Geometry: final body of the model. Coordinates: model frame, mm. Face numbers are marked on the shaded views. A direction names the side the tool comes from. Coordinates: 2 decimals unless noted, no trailing zeros. Order: outer loops, then holes, each group sorted by start corner. A loop starts at its lowest first (then second) coordinate and runs counter-clockwise, first axis right, second up. Notation, with made-up numbers: (-21, -16) - (10, -16) arc R17 ccw to (10, 13) - close; hole circle Ø9 at (9, 68). An arc over 180 degrees is marked (long way). Use a Markdown table: item, result. Add a question column.
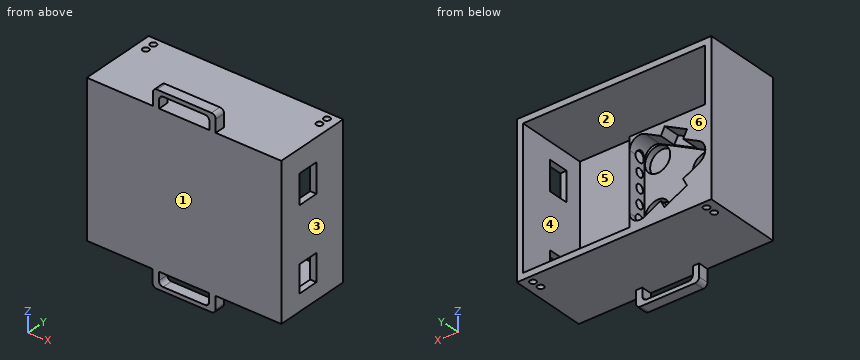
```python
from build123d import *

# Parameters (mm, degrees)
SKETCH1_W           = 92.7
SKETCH1_H           = 37
BOSS_EXTRUDE1_DEPTH = 72
SKETCH3_W           = 86.7
SKETCH3_H           = 66
CUT_EXTRUDE1_DEPTH  = 34
SKETCH6_W           = 13
SKETCH6_H           = 10
SKETCH6_W_2         = 14
CUT_EXTRUDE2_DEPTH  = 3
SKETCH8_W           = 30
SKETCH8_H           = 5
BOSS_EXTRUDE2_DEPTH = 8
SKETCH9_W           = 24
SKETCH9_H           = 6
CUT_EXTRUDE3_DEPTH  = 8
FILLET3_R           = 2
FILLET4_R           = 2
SKETCH10_W          = 30
SKETCH10_H          = 5
BOSS_EXTRUDE3_DEPTH = 8
SKETCH11_W          = 24
SKETCH11_H          = 6
CUT_EXTRUDE4_DEPTH  = 8
FILLET5_R           = 2
BOSS_EXTRUDE4_DEPTH = 40
CUT_EXTRUDE5_DEPTH  = 9
SKETCH15_R          = 6
CUT_EXTRUDE6_DEPTH  = 12
CUT_EXTRUDE7_DEPTH  = 8
SKETCH26_R          = 2.5
SKETCH26_R_2        = 2
CUT_EXTRUDE8_DEPTH  = 1


with BuildPart() as part:
    # Sketch1 → Boss-Extrude1 (new body)
    with BuildSketch(Plane.XY):
        with Locations((46.35, 18.5)):
            Rectangle(SKETCH1_W, SKETCH1_H)
    extrude(amount=-BOSS_EXTRUDE1_DEPTH)

    # Sketch3 → Cut-Extrude1 (cut)
    with BuildSketch(Plane(origin=(0, 37, 0), x_dir=(1, 0, 0), z_dir=(0, 1, 0))):
        with Locations((46.35, 36)):
            Rectangle(SKETCH3_W, SKETCH3_H)
    extrude(amount=-CUT_EXTRUDE1_DEPTH, mode=Mode.SUBTRACT)

    # Sketch6 → Cut-Extrude2 (cut)
    with BuildSketch(Plane(origin=(92.7, 0, 0), x_dir=(0, 0, -1), z_dir=(1, 0, 0))):
        with Locations((57.5, 16)):
            Rectangle(SKETCH6_W, SKETCH6_H)
        with Locations((18, 16)):
            Rectangle(SKETCH6_W_2, SKETCH6_H)
    extrude(amount=-CUT_EXTRUDE2_DEPTH, mode=Mode.SUBTRACT)

    # Sketch8 → Boss-Extrude2 (add)
    with BuildSketch(Plane.XY):
        with Locations((46.447728755, 2.5)):
            Rectangle(SKETCH8_W, SKETCH8_H)
    extrude(amount=BOSS_EXTRUDE2_DEPTH)

    # Sketch9 → Cut-Extrude3 (cut)
    with BuildSketch(Plane(origin=(0, 5, 0), x_dir=(1, 0, 0), z_dir=(0, 1, 0))):
        with Locations((46.447728755, -3)):
            Rectangle(SKETCH9_W, SKETCH9_H)
    extrude(amount=-CUT_EXTRUDE3_DEPTH, mode=Mode.SUBTRACT)

    # Fillet3
    fillet3_edges = [part.edges().sort_by_distance(p)[0] for p in [
        (31.447728755, 2.5, 8),
        (61.447728755, 2.5, 8),
    ]]
    fillet(fillet3_edges, radius=FILLET3_R)

    # Fillet4
    fillet4_edges = [part.edges().sort_by_distance(p)[0] for p in [
        (58.447728755, 2.5, 6),
        (34.447728755, 2.5, 6),
    ]]
    fillet(fillet4_edges, radius=FILLET4_R)

    # Sketch10 → Boss-Extrude3 (add)
    with BuildSketch(Plane(origin=(0, 0, -72), x_dir=(-1, 0, 0), z_dir=(0, 0, -1))):
        with Locations((-46.35, 2.5)):
            Rectangle(SKETCH10_W, SKETCH10_H)
    extrude(amount=BOSS_EXTRUDE3_DEPTH)

    # Sketch11 → Cut-Extrude4 (cut)
    with BuildSketch(Plane(origin=(0, 5, 0), x_dir=(1, 0, 0), z_dir=(0, 1, 0))):
        with Locations((46.35, 75)):
            Rectangle(SKETCH11_W, SKETCH11_H)
    extrude(amount=-CUT_EXTRUDE4_DEPTH, mode=Mode.SUBTRACT)

    # Fillet5
    fillet5_edges = [part.edges().sort_by_distance(p)[0] for p in [
        (61.35, 2.5, -80),
        (31.35, 2.5, -80),
        (34.35, 2.5, -78),
        (58.35, 2.5, -78),
    ]]
    fillet(fillet5_edges, radius=FILLET5_R)

    # Sketch13 → Boss-Extrude4 (add)
    with BuildSketch(Plane.XY.offset(-69)):
        Polygon((3, 37), (3, 25), (16, 25), (16, 26), (26, 26), (26, 25), (39, 25), (39, 37), align=None)
    extrude(amount=BOSS_EXTRUDE4_DEPTH)

    # Sketch14 → Cut-Extrude5 (cut)
    with BuildSketch(Plane(origin=(0, 37, 0), x_dir=(1, 0, 0), z_dir=(0, 1, 0))):
        with BuildLine():
            Line((31.604139479, 30.654513564), (5.825726754, 44.05502325))
            ThreePointArc((5.825726754, 44.05502325), (2.862548541, 48.948836401), (5.850230218, 53.827728742))
            Line((5.850230218, 53.827728742), (31.695517579, 67.098800427))
            ThreePointArc((31.695517579, 67.098800427), (36.590581321, 66.914928251), (38.979411894, 62.638370465))
            Line((38.979411894, 62.638370465), (38.91030967, 35.078361321))
            ThreePointArc((38.91030967, 35.078361321), (36.500063726, 30.813836436), (31.604139479, 30.654513564))
        make_face()
    extrude(amount=-CUT_EXTRUDE5_DEPTH, mode=Mode.SUBTRACT)

    # Sketch15 → Cut-Extrude6 (cut)
    with BuildSketch(Plane(origin=(0, 28, 0), x_dir=(1, 0, 0), z_dir=(0, 1, 0))):
        with Locations(Location((32.730960784, 37.059306593, 0), (0, 0, 270))):
            Circle(SKETCH15_R)
        with Locations(Location((32.730960784, 60.777824087, 0), (0, 0, 270))):
            Circle(SKETCH15_R)
        with Locations(Location((9.931562791, 48.935046092, 0), (0, 0, 270))):
            Circle(SKETCH15_R)
    extrude(amount=-CUT_EXTRUDE6_DEPTH, mode=Mode.SUBTRACT)

    # Sketch17 → Cut-Extrude7 (cut)
    with BuildSketch(Plane(origin=(0, 37, 0), x_dir=(1, 0, 0), z_dir=(0, 1, 0))):
        Polygon((18.772873899, 60.463264585), (24.11034588, 63.203956622), (22.283217855, 66.762271277), (11.608273892, 61.280887201), (13.435401917, 57.722572547), align=None)
        Polygon((18.714933117, 37.354768407), (24.038594399, 34.587345318), (22.193645673, 31.038237797), (11.546323109, 36.573083975), (13.391271835, 40.122191496), align=None)
    extrude(amount=-CUT_EXTRUDE7_DEPTH, mode=Mode.SUBTRACT)

    # Sketch20 → Cut-Revolve1 (revolve, cut)
    with BuildSketch(Plane.XY):
        with BuildLine():
            Line((5, 32), (5, 35))
            ThreePointArc((5, 35), (3.5, 33.5), (5, 32))
        make_face()
        with BuildLine():
            Line((5, 27.5), (5, 30.5))
            ThreePointArc((5, 30.5), (3.5, 29), (5, 27.5))
        make_face()
    revolve(axis=Axis((5, 32, 0), (0, 1, 0)), mode=Mode.SUBTRACT)

    # Sketch22 → Cut-Revolve2 (revolve, cut)
    with BuildSketch(Plane.XY):
        with BuildLine():
            Line((87.7, 35), (87.7, 32))
            ThreePointArc((87.7, 32), (86.2, 33.5), (87.7, 35))
        make_face()
        with BuildLine():
            Line((87.7, 30.5), (87.7, 27.5))
            ThreePointArc((87.7, 27.5), (86.2, 29), (87.7, 30.5))
        make_face()
    revolve(axis=Axis((87.7, 35, 0), (0, -1, 0)), mode=Mode.SUBTRACT)

    # Sketch23 → Cut-Revolve8 (revolve, cut)
    with BuildSketch(Plane(origin=(0, 0, -72), x_dir=(-1, 0, 0), z_dir=(0, 0, -1))):
        with BuildLine():
            Line((-87.7, 35), (-87.7, 32))
            ThreePointArc((-87.7, 32), (-89.2, 33.5), (-87.7, 35))
        make_face()
        with BuildLine():
            Line((-87.7, 30.5), (-87.7, 27.5))
            ThreePointArc((-87.7, 27.5), (-89.2, 29), (-87.7, 30.5))
        make_face()
    revolve(axis=Axis((87.7, 35, -72), (0, -1, 0)), mode=Mode.SUBTRACT)

    # Sketch24 → Cut-Revolve9 (revolve, cut)
    with BuildSketch(Plane(origin=(0, 0, -72), x_dir=(-1, 0, 0), z_dir=(0, 0, -1))):
        with BuildLine():
            Line((-5, 35), (-5, 32))
            ThreePointArc((-5, 32), (-6.5, 33.5), (-5, 35))
        make_face()
        with BuildLine():
            Line((-5, 27.5), (-5, 30.5))
            ThreePointArc((-5, 30.5), (-6.5, 29), (-5, 27.5))
        make_face()
    revolve(axis=Axis((5, 35, -72), (0, -1, 0)), mode=Mode.SUBTRACT)

    # Sketch26 → Cut-Extrude8 (cut)
    with BuildSketch(Plane(origin=(39, 0, 0), x_dir=(0, 0, -1), z_dir=(1, 0, 0))):
        with Locations((63, 31)):
            Circle(SKETCH26_R)
        with Locations((56, 31)):
            Circle(SKETCH26_R_2)
        with BuildLine():
            ThreePointArc((49, 33), (47, 31), (49, 29))
            Line((49, 29), (49, 33))
        make_face()
        with BuildLine():
            Line((49, 33), (49, 29))
            ThreePointArc((49, 29), (50.414213562, 29.585786438), (51, 31))
            ThreePointArc((51, 31), (50.414213562, 32.414213562), (49, 33))
        make_face()
        with Locations((42, 31)):
            Circle(SKETCH26_R_2)
        with Locations((35, 31)):
            Circle(SKETCH26_R)
    extrude(amount=-CUT_EXTRUDE8_DEPTH, mode=Mode.SUBTRACT)


solid = part.part
```
1) First-contact query: pin 1 (6 mm diameter, centred on x = 71, y = 18.5, fed in from +Z); pin 2 (17 mm diameter, centred on x = 31, y = 28, fed in from -Z); pin 3 (4 mm diameter, centred on x = 37, z = -15.5, fed in from +Y). Flat tips, straight axial feed; report the tip coordinate or a pass-through.
2) Section query C-C (x = 49.5). Return the cut outline in (y, z), and give its area (3 significant figures).
3) Section query A-A (z = -18). Return the cut outline in (x, y), and give its area (3 significant figures).
4) Section query B-B (y = 18.5). Return the cut outline in (x, z), and give its area (3 significant figures).
5) Line query: line 1 (Z direction, x = 38.75, y = 31); line 2 (X direction, y = 6, z = -53.5); line 3 (Z direction, x = 73.5, y = 26.5). Output: solid intervals per line, ascending. Write a range as from..to.
6) Draft query along X for the marked faces 1, 2 and 3. Return one class per face: released by +X, released by -X, zero draft, split by the parting line, or undercut.
7) Section query D-D (x = 63.5). Return the cut outline in (y, z), and give its area (3 significant figures).
8) Access query for the marked faces 4, 5 and 6. Directions: +Z, -Z, +X, -X, +Y, -Y. A direction counts if a zero-diameter tool reaches every point of the face in a straight line with its end or side. Return the directions, or none.
From the geometry:
| question | item | result |
|---|---|---|
| 1 | pin 1 | stops at z = 0 |
| 1 | pin 2 | stops at z = -72 |
| 1 | pin 3 | stops at y = 3 |
| 2 | outline | (0, -80) - (5, -80) - (5, -78) - (0, -78) - close; (0, -72) - (37, -72) - (37, -69) - (3, -69) - (3, -3) - (37, -3) - (37, 0) - (0, 0) - close; (0, 6) - (5, 6) - (5, 8) - (0, 8) - close |
| 2 | area | 440 mm^2 |
| 3 | outline | (0, 0) - (92.7, 0) - (92.7, 11) - (89.7, 11) - (89.7, 3) - (3, 3) - (3, 37) - (0, 37) - close; (89.7, 21) - (92.7, 21) - (92.7, 37) - (89.7, 37) - close |
| 3 | area | 452 mm^2 |
| 4 | outline | (0, -72) - (92.7, -72) - (92.7, -64) - (89.7, -64) - (89.7, -69) - (3, -69) - (3, -3) - (89.7, -3) - (89.7, -11) - (92.7, -11) - (92.7, 0) - (0, 0) - close; (89.7, -51) - (92.7, -51) - (92.7, -25) - (89.7, -25) - close |
| 4 | area | 871 mm^2 |
| 5 | line 1 | z = -72..-65.5, -32.5..-29, -3..0 |
| 5 | line 2 | x = 0..3, 89.7..92.7 |
| 5 | line 3 | z = -72..-69, -3..0 |
| 6 | face 1 | zero draft |
| 6 | face 2 | undercut |
| 6 | face 3 | released by +X |
| 7 | outline | (0, -72) - (37, -72) - (37, -69) - (3, -69) - (3, -3) - (37, -3) - (37, 0) - (0, 0) - close |
| 7 | area | 420 mm^2 |
| 8 | face 4 | +Y |
| 8 | face 5 | none |
| 8 | face 6 | +Z, -Z, +X, -X, +Y |
